Could you check a few things on this model? Use its own coordinates, in mm. A direction names the side the tool comes from. Round coordinates to 2 decimals unless told otherwise and drop trailing zeros. Write each loop counter-clockwise with the first axis right and the second up, starting at its lowest first coordinate (ties: lowest second). Pieces come first, ordered by that corner, then holes. Notation, with made-up numbers: (44.25, 38) -> (87.25, 38) arc R27 ccw to (87.25, 59) -> close; hole circle Ø3 at (2, 0.25). An arc over 180 degrees is marked (long way). Return JSON: item names as keys, results as strings.
from build123d import *

# Parameters (mm, degrees)
SKETCH_W              = 150
SKETCH_H              = 25
PAD_DEPTH             = 3
PAD001_DEPTH          = 3
SKETCH004_W           = 150
SKETCH004_H           = 25
SKETCH004_W_2         = 96
SKETCH004_H_2         = 2.9
PAD002_DEPTH          = 3
SKETCH005_R           = 0.85
POCKET_DEPTH          = 313.671314
POLARPATTERN_COUNT    = 2
POLARPATTERN001_COUNT = 2
POLARPATTERN002_COUNT = 2
FILLET_R              = 5


with BuildPart() as part:
    # Sketch → Pad (new body)
    with BuildSketch(Plane.XY):
        Rectangle(SKETCH_W, SKETCH_H)
    extrude(amount=PAD_DEPTH)

    # Sketch001 (on Face6 of Pad) → Pad001 (join)
    with BuildSketch(Plane.XY.offset(3)):
        Polygon((-75, 12.5), (75, 12.5), (75, 4), (50, 4), (50, 5), (-50, 5), (-50, 4), (-52.25, 4), (-52.25, 9.2), (-72.25, 9.2), (-72.25, 4.5), (-75, 4.5), align=None)
        Polygon((-75, -12.5), (75, -12.5), (75, -4), (50, -4), (50, -5), (-50, -5), (-50, -4), (-52.25, -4), (-52.25, -9.2), (-72.25, -9.2), (-72.25, -4.5), (-75, -4.5), align=None)
    extrude(amount=PAD001_DEPTH)

    # Sketch004 (on Face12 of Pad001) → Pad002 (join)
    with BuildSketch(Plane.XY.offset(6)):
        Rectangle(SKETCH004_W, SKETCH004_H)
        Rectangle(SKETCH004_W_2, SKETCH004_H_2, mode=Mode.SUBTRACT)
    extrude(amount=PAD002_DEPTH)

    # Sketch005 (on Face34 of Pad002) → Pocket (cut, through all)
    with BuildSketch(Plane.XY.offset(9)):
        with Locations((-70, 7.5)):
            Circle(SKETCH005_R)
    pocket = extrude(amount=-POCKET_DEPTH, mode=Mode.SUBTRACT)

    # PolarPattern: Pocket ×2 about axis
    polarpattern_axis = Axis((0, 0, 9), (0, 0, 1))
    for i in range(1, POLARPATTERN_COUNT):
        add(pocket.rotate(polarpattern_axis, i * 360 / POLARPATTERN_COUNT), mode=Mode.SUBTRACT)

    # PolarPattern001: Pocket ×2 about axis
    polarpattern001_axis = Axis((0, 0, 0), (0, 1, 0))
    for i in range(1, POLARPATTERN001_COUNT):
        add(pocket.rotate(polarpattern001_axis, i * 360 / POLARPATTERN001_COUNT), mode=Mode.SUBTRACT)

    # PolarPattern002: Pocket ×2 about axis
    polarpattern002_axis = Axis((0, 0, 0), (1, 0, 0))
    for i in range(1, POLARPATTERN002_COUNT):
        add(pocket.rotate(polarpattern002_axis, i * 360 / POLARPATTERN002_COUNT), mode=Mode.SUBTRACT)

    # Fillet
    fillet_edges = [part.edges().sort_by_distance(p)[0] for p in [
        (75, -12.5, 7.5),
        (75, 12.5, 7.5),
        (-75, -12.5, 7.5),
        (-75, 12.5, 7.5),
    ]]
    fillet(fillet_edges, radius=FILLET_R)


solid = part.part
1) Thinking about a two-plate mould opening in Z: for faces 4 (the face through (-1, 3, 9)), 5 (the face through (-72.25, 7, 4)), 6 (the face through (-1, -1.45, 7)), 7 (the face through (-74, 4.5, 4)), which applies, pulls with the +Z half, pulls with the -Z half, needs draft (parallel to the pull), parting line crosses it, or undercut?
Return value:
{"face 4": "pulls with the +Z half", "face 5": "undercut", "face 6": "needs draft", "face 7": "undercut"}
2) I want a section at A-A, the plane z = 4.5. Count the separate pieces of the cut face and the enclosed holes in it, and give its area (3 significant figures).
Return value:
{"separate pieces": "2", "enclosed holes": "2", "area": "2,110 mm²"}
3) Will this pin go through, and if not, where does the flat tip stop? pin 1 Ø2 at (x, z) = (-74, 5) entering from -Y.
Return value:
{"pin 1": "y = -11.5"}
4) I want a section at C-C, the plane x = 16.5. Please give me the cut outline in (y, z), and give its area (3 significant figures).
Return value:
{"outline": "(-12.5, 0) -> (12.5, 0) -> (12.5, 9) -> (1.45, 9) -> (1.45, 6) -> (5, 6) -> (5, 3) -> (-5, 3) -> (-5, 6) -> (-1.45, 6) -> (-1.45, 9) -> (-12.5, 9) -> close", "area": "186 mm²"}
5) If I drill on probe 1 along Y at (x, z) = (-70, 0.8); probe 2 along Y at (x, z) = (40, 4); probe 3 along X at (y, z) = (-7.5, 0.7), over which ranges is the centre line in solid material (lowest first)? Write a range as [from, to].
Return value:
{"probe 1": "[-12.5, -8.35], [-6.65, 6.65], [8.35, 12.5]", "probe 2": "[-12.5, -5], [5, 12.5]", "probe 3": "[-75, -70.85], [-69.15, 69.15], [70.85, 75]"}
6) I want a section at B-B, the plane y = -2.75. Please give me the cut outline in (x, z), and give its area (3 significant figures).
Return value:
{"outline": "(-75, 0) -> (75, 0) -> (75, 3) -> (-75, 3) -> close; (-75, 6) -> (75, 6) -> (75, 9) -> (-75, 9) -> close", "area": "900 mm²"}
7) For faces 1 (the face through (-62, -9.2, 4)), 2 (the face through (48, 0, 7)), 3 (the face through (63, 4, 4)), which set-ups out of +Z, -Z, +X, -X, +Y, -Y let a thin tool reach every point of the face, with its end or its side?
Return value:
{"face 1": "none", "face 2": "+Z", "face 3": "+X, -X"}
